from build123d import *

# Parameters (mm, degrees)
F0_W     = 60
F0_H     = 67.5
F1_DEPTH = 15
F3_DEPTH = 3


with BuildPart() as f1:
    # F0 (on Top) → F1 (new body)
    with BuildSketch(Plane.XY):
        with Locations((-30, 33.75)):
            Rectangle(F0_W, F0_H)
        Polygon((60, 67.5), (0, 67.5), (0, 0), (5.978101, 0), (60, 0), align=None)
        with Locations((-30, -33.75)):
            Rectangle(F0_W, F0_H)
        Polygon((5.978101, 0), (0, 0), (0, -67.5), (60, -67.5), (60, 0), align=None)
    extrude(amount=F1_DEPTH)

    # F2 (on face) → F3 (join)
    with BuildSketch(Plane.XY.offset(15)):
        Polygon((9.656936, 0), (30.810218, 17.819343), (50.12409, 0), (58.597274, 0), (30.810218, 25.636863), (0.376784, 0), align=None)
        Polygon((0.376784, 20.34854), (0.376784, 9.886861), (30.810218, 35.523724), (60, 9.569461), (60, 18.968979), (30.810218, 45.985403), align=None)
        Polygon((0.376784, 43.571167), (0.376784, 31.844892), (30.810218, 57.481755), (60, 31.155111), (60, 41.173357), (30.810218, 67.5), align=None)
    extrude(amount=F3_DEPTH)


solid = f1.part
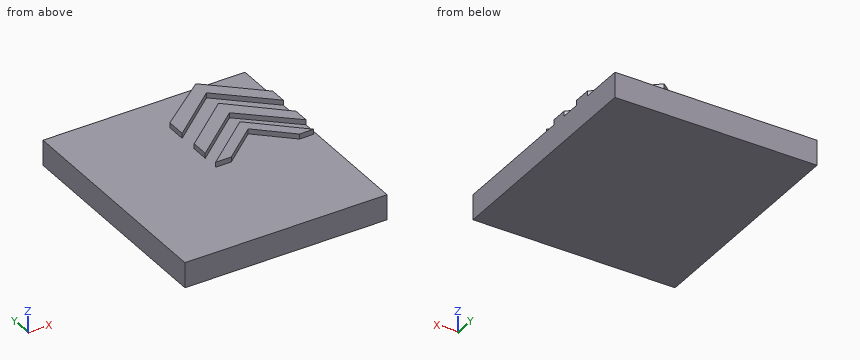
Input: part model. Units: mm. Frame: model coordinates. Give positions to 0.01 mm unless a question says otherwise; leave off trailing zeros. Write each loop counter-clockwise with the first axis right and the second up, starting at its lowest first coordinate (ties: lowest second). Pieces come first, ordered by that corner, then holes.
Q1. Section A-A, the plane y = 16. Output: boundary loops of the cut face in (x, z).
Q2. Material intervals for probe 1 along X at (y, z) = (17, 16.5); probe 2 along Z at (x, y) = (-15, -23), sorted ascending.
Q3. Section D-D, the plane y = -37.5. Output: boundary loops of the cut face in (x, z).
Q4. Section C-C, the plane x = 46. Output: boundary loops of the cut face in (y, z).
Q5. First-contact query: P1, Ø3.5, axis at y = 16, z = 17, coming from the -X side; P2, Ø2.5, axis at x = 55.5, z = 17, coming from the -Y side. Flat tips, straight axial feed; report the tip coordinate or a pass-through.
Q6. Section B-B, the plane x = 2.5. Output: boundary loops of the cut face in (y, z), plus the area to 3 significant figures.
Filled in:
1. outline: (-60, 0) - (60, 0) - (60, 18) - (52.77, 18) - (52.77, 15) - (41.26, 15) - (41.26, 18) - (32.78, 18) - (32.78, 15) - (28.65, 15) - (28.65, 18) - (19.37, 18) - (19.37, 15) - (7.63, 15) - (7.63, 18) - (0.38, 18) - (0.38, 15) - (-60, 15) - close
2. probe 1: x = 0.38 to 8.82, 20.56 to 29.84, 31.7 to 40.17, 51.64 to 60
2. probe 2: z = 0 to 15
3. outline: (-60, 0) - (60, 0) - (60, 15) - (-60, 15) - close
4. outline: (-67.5, 0) - (67.5, 0) - (67.5, 15) - (53.8, 15) - (53.8, 18) - (43.78, 18) - (43.78, 15) - (31.93, 15) - (31.93, 18) - (22.02, 18) - (22.02, 15) - (11.62, 15) - (11.62, 18) - (3.8, 18) - (3.8, 15) - (-67.5, 15) - close
5. P1: stops at x = 0.38
5. P2: stops at y = 0
6. outline: (-67.5, 0) - (67.5, 0) - (67.5, 15) - (45.24, 15) - (45.24, 18) - (33.63, 18) - (33.63, 15) - (22.14, 15) - (22.14, 18) - (11.68, 18) - (11.68, 15) - (1.79, 15) - (1.79, 18) - (0, 18) - (0, 15) - (-67.5, 15) - close
6. area: 2,100 mm2
